```python
from build123d import *

# Parameters (mm, degrees)
SKETCH1_R           = 50
BOSS_EXTRUDE1_DEPTH = 10
SKETCH2_R           = 15
BOSS_EXTRUDE2_DEPTH = 25
SKETCH3_W           = 60
SKETCH3_H           = 3
BOSS_EXTRUDE3_DEPTH = 70
SKETCH4_R           = 10
BOSS_EXTRUDE4_DEPTH = 63


with BuildPart() as part:
    # Sketch1 → Boss-Extrude1 (new body)
    with BuildSketch(Plane(origin=(0, 0, 0), x_dir=(1, 0, 0), z_dir=(0, 1, 0))):
        with Locations(Location((0, 0, 0), (0, 0, 270))):
            Circle(SKETCH1_R)
    extrude(amount=BOSS_EXTRUDE1_DEPTH)

    # Sketch2 → Boss-Extrude2 (add)
    with BuildSketch(Plane(origin=(0, 0, 0), x_dir=(-1, 0, 0), z_dir=(0, -1, 0))):
        with Locations(Location((0, 0, 0), (0, 0, 90))):
            Circle(SKETCH2_R)
    extrude(amount=BOSS_EXTRUDE2_DEPTH)

    # Sketch3 → Boss-Extrude3 (add)
    with BuildSketch(Plane(origin=(0, 10, 0), x_dir=(1, 0, 0), z_dir=(0, 1, 0))):
        with Locations((0, -31.5)):
            Rectangle(SKETCH3_W, SKETCH3_H)
        with Locations((0, 31.5)):
            Rectangle(SKETCH3_W, SKETCH3_H)
    extrude(amount=BOSS_EXTRUDE3_DEPTH)

    # Sketch4 → Boss-Extrude4 (add)
    with BuildSketch(Plane.XY.offset(33)):
        with Locations((0, 61.110810205)):
            Circle(SKETCH4_R)
    extrude(amount=-BOSS_EXTRUDE4_DEPTH)


solid = part.part
```
Verification items for the finished model (mm, model axes). A direction names the side the tool comes from. Round coordinates to 2 decimals unless told otherwise and drop trailing zeros. Order: outer loops, then holes, each group sorted by start corner. A loop starts at its lowest first (then second) coordinate and runs counter-clockwise, first axis right, second up. Notation, with made-up numbers: (-25.5, 83) - (-11.5, 83) arc R32 ccw to (-11.5, 118) - close; hole circle Ø3 at (-32, 53). An arc over 180 degrees is marked (long way). Use CSV: the item, a comma, the result in double quotes. Start each with the question number.
1) Go/stop test with flat-tipped pins: P1, Ø3.5, axis at y = 62, z = 31, coming from the +X side; P2, Ø2.5, axis at y = 60, z = -32, coming from the -X side; P3, Ø12, axis at y = 53.5, z = 10, coming from the -X side. Record where each tip stops, or that it passes through.
2) Section check C-C, the plane z = 4. Record the cut outline in (x, y), plus the area to 3 significant figures.
3) Section check A-A, the plane x = 0. Record the cut outline in (y, z), plus the area to 3 significant figures.
4) Thickness scan on L1, parallel to Z at x = -10, y = 16.5; L2, parallel to Y at x = -46, z = 9; L3, parallel to Y at x = 9, z = 3. Record the ranges inside material, lowest first.
5) Access from +Z, -Z, +X, -X, +Y, -Y to the whole of each face (thin tool, end or side, straight path). Record for faces 4 (the flat face through (0, 45, -33)), 5 (the flat face through (-30, 45, -31)), 6 (the cylindrical face through (0.66, -12.325, 14.985)).
6) Mould release check, pull along Z, two halves, no side actions. Record for faces 1 (the flat face through (0, 45, 30)), 2 (the flat face through (-30, 45, 32)), 3 (the flat face through (0, 45, 33)): +Z half, -Z half, draft (parallel to the pull), parting line (faces both ways), or undercut.
7) Section check D-D, the plane x = -21. Record the cut outline in (y, z), plus the area to 3 significant figures.
8) Section check B-B, the plane y = 44.5. Record the cut outline in (x, z), plus the area to 3 significant figures.
Answers:
1,P1,"stops at x = 30"
1,P2,"stops at x = -30"
1,P3,"stops at x = -9.87"
2,outline,"(-49.84, 0) - (-14.46, 0) - (-14.46, -25) - (14.46, -25) - (14.46, 0) - (49.84, 0) - (49.84, 10) - (-49.84, 10) - close; circle Ø20 at (0, 61.11)"
2,area,"2,030 mm²"
3,outline,"(-25, -15) - (0, -15) - (0, -50) - (10, -50) - (10, -33) - (80, -33) - (80, -30) - (71.11, -30) - (71.11, 30) - (80, 30) - (80, 33) - (10, 33) - (10, 50) - (0, 50) - (0, 15) - (-25, 15) - close; hole (10, -30) - (51.11, -30) - (51.11, 30) - (10, 30) - close"
3,area,"3,370 mm²"
4,L1,"z = -33 to -30, 30 to 33"
4,L2,"y = 0 to 10"
4,L3,"y = -25 to 10, 56.75 to 65.47"
5,face 4,"-Z, +X, -X, +Y"
5,face 5,"+Z, -Z, -X, +Y"
5,face 6,"-Y"
6,face 1,"undercut"
6,face 2,"draft"
6,face 3,"+Z half"
7,outline,"(0, -45.38) - (10, -45.38) - (10, -33) - (80, -33) - (80, -30) - (10, -30) - (10, 30) - (80, 30) - (80, 33) - (10, 33) - (10, 45.38) - (0, 45.38) - close"
7,area,"1,330 mm²"
8,outline,"(-30, -33) - (30, -33) - (30, -30) - (-30, -30) - close; (-30, 30) - (30, 30) - (30, 33) - (-30, 33) - close"
8,area,"360 mm²"
